The model under review builds one solid part; all positions refer to its coordinate system, in mm. Coordinates: 2 decimals unless noted, no trailing zeros. Write each loop counter-clockwise with the first axis right and the second up, starting at its lowest first coordinate (ties: lowest second). Pieces come first, ordered by that corner, then holes.
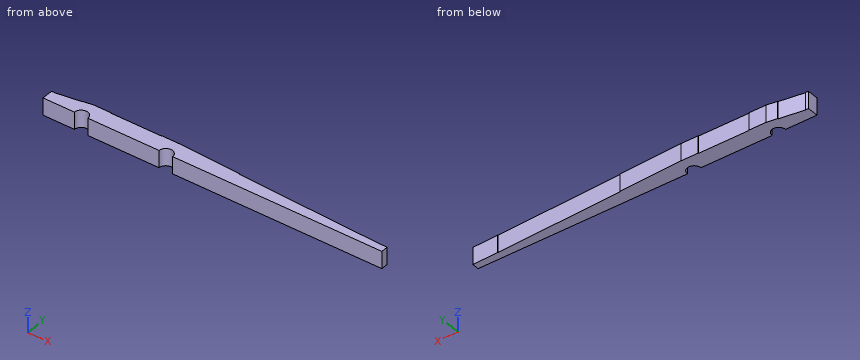
```python
from build123d import *

# Parameters (mm, degrees)
BOSS_EXTRUDE1_DEPTH = 20
SKETCH2_W           = 150
SKETCH2_H           = 20
ROPEGROOVE1_DEPTH   = 0.5
SKETCH4_W           = 60
SKETCH4_H           = 20
ROPEGROOVE2_DEPTH   = 0.5
SKETCH5_W           = 30
SKETCH5_H           = 20
ROPEGROOVE3_DEPTH   = 0.5


with BuildPart() as part:
    # Sketch1 → Boss-Extrude1 (new body)
    with BuildSketch(Plane.XY):
        with BuildLine():
            Line((-8, 0), (-92, 0))
            ThreePointArc((-92, 0), (-100, 8), (-108, 0))
            Line((-108, 0), (-145, 0))
            Line((-145, 0), (-145, 13))
            Line((-145, 13), (-100, 20))
            Line((-100, 20), (0, 20))
            Line((0, 20), (255, 8))
            Line((255, 8), (255, 0))
            Line((255, 0), (8, 0))
            ThreePointArc((8, 0), (0, 8), (-8, 0))
        make_face()
    extrude(amount=BOSS_EXTRUDE1_DEPTH)

    # Sketch2 → RopeGroove1 (cut)
    with BuildSketch(Plane(origin=(0.93909681, 19.955807209, 0), x_dir=(0.9988945692351382, -0.047006803258124105, 0), z_dir=(0.047006803258124105, 0.9988945692351382, 0))):
        with Locations((149.059863935, -10)):
            Rectangle(SKETCH2_W, SKETCH2_H)
    extrude(amount=-ROPEGROOVE1_DEPTH, mode=Mode.SUBTRACT)

    # Sketch4 → RopeGroove2 (cut)
    with BuildSketch(Plane(origin=(0, 20, 0), x_dir=(1, 0, 0), z_dir=(0, 1, 0))):
        with Locations((-50, -10)):
            Rectangle(SKETCH4_W, SKETCH4_H)
    extrude(amount=-ROPEGROOVE2_DEPTH, mode=Mode.SUBTRACT)

    # Sketch5 → RopeGroove3 (cut)
    with BuildSketch(Plane(origin=(-5.400192864, 34.715525554, 0), x_dir=(0.9881164689548824, 0.15370700628187053, 0), z_dir=(-0.15370700628187053, 0.9881164689548824, 0))):
        with Locations((-123.278696917, -10)):
            Rectangle(SKETCH5_W, SKETCH5_H)
    extrude(amount=-ROPEGROOVE3_DEPTH, mode=Mode.SUBTRACT)


solid = part.part
```
Item 1: Take a section at A-A, the plane y = 5. Write out the cut boundary in (x, z) (3 decimals), plus the area to 3 significant figures.
Solved:
outline: (-145, 0) - (-106.245, 0) - (-106.245, 20) - (-145, 20) - close; (-93.755, 0) - (-6.245, 0) - (-6.245, 20) - (-93.755, 20) - close; (6.245, 0) - (255, 0) - (255, 20) - (6.245, 20) - close
area: 7,500 mm2
Item 2: Take a section at B-B, the plane z = 10.25. Write out the cut boundary in (x, y), plus the area to 3 significant figures.
Solved:
outline: (-145, 0) - (-108, 0) arc R8 cw to (-92, 0) - (-8, 0) arc R8 cw to (8, 0) - (255, 0) - (255, 8) - (224.75, 9.42) - (224.73, 8.92) - (74.89, 15.98) - (74.92, 16.47) - (0, 20) - (-20, 20) - (-20, 19.5) - (-80, 19.5) - (-80, 20) - (-100, 20) - (-112.39, 18.07) - (-112.32, 17.58) - (-141.96, 12.97) - (-142.04, 13.46) - (-145, 13) - close
area: 5,990 mm2
Item 3: Take a section at D-D, the plane x = 82. Write out the cut boundary in (y, z).
Solved:
outline: (0, 0) - (15.64, 0) - (15.64, 20) - (0, 20) - close
Item 4: Take a section at C-C, the plane x = -67. Write out the cut boundary in (y, z).
Solved:
outline: (0, 0) - (19.5, 0) - (19.5, 20) - (0, 20) - close
Item 5: To check wall thickness, follow line 1 along X through (y, z) = (6, 11); line 2 along Y through (x, z) = (-63, 4.5); line 3 along Y through (x, z) = (215.5, 9). State the ranges of each line that lie inside material, in increasing order.
Solved:
line 1: x = -145 to -105.29, -94.71 to -5.29, 5.29 to 255
line 2: y = 0 to 19.5
line 3: y = 0 to 9.36
Item 6: For pin 1 (1.5 mm diameter, centred on x = 6.5, z = 13, fed in from -Y); pin 2 (12 mm diameter, centred on x = 180.5, z = 16.5, fed in from +Y); pin 3 (12 mm diameter, centred on x = 119, z = 9, fed in from +Y), all flat-tipped, find the tip position at first contact; note any pin that passes through.
Solved:
pin 1: stops at y = 3.38
pin 2: stops at y = 11.29
pin 3: stops at y = 14.18
